Design review of the part built by this model. Coordinates are the model's own, in mm. Face numbers are marked on the shaded views. Give positions to 0.01 mm unless a question says otherwise; leave off trailing zeros. Loops run counter-clockwise (first coordinate to the right, second up) from the corner with the lowest first, then second, coordinate; pieces in that order, holes last. Notation, with made-up numbers: (2.5, 83.5) -> (46.5, 83.5) arc R17 ccw to (46.5, 96.5) -> close; hole circle Ø8 at (18.5, 63.25). An arc over 180 degrees is marked (long way). Use a Markdown table: item, result. Add a question column.
1. Add section B-B (z = 4). State the section outline as (x, y) points (3 decimals).
2. To check wall thickness, follow line 1 (X direction, y = -40.5, z = 4.25); line 2 (Y direction, x = -30.5, z = 2.75); line 3 (X direction, y = 5.5, z = 2.75). State the ranges of each line that lie inside material, in increasing order.
3. Add section C-C (y = 38.5). State the section outline as (x, z) points, and give its area (3 significant figures).
4. Add section A-A (x = 36.5). State the section outline as (y, z) points, and give its area (3 significant figures).
5. Draft analysis for pull direction Y (two halves, no side actions). For the marked faces 1 and 2, state which applies: pulls with the +Y half, pulls with the -Y half, needs draft (parallel to the pull), parting line crosses it, or undercut.
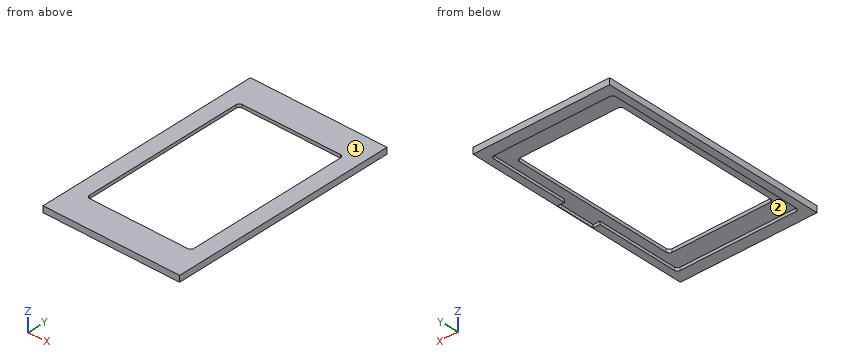
```python
from build123d import *

# Parameters (mm, degrees)
SKETCH1_W           = 140
SKETCH1_H           = 234
BOSS_EXTRUDE1_DEPTH = 6.35
SKETCH2_W           = 107
SKETCH2_H           = 172
CUT_EXTRUDE1_DEPTH  = 137.489276136
FILLET1_R           = 3.175
SKETCH3_W           = 125
SKETCH3_H           = 210
CUT_EXTRUDE2_DEPTH  = 3
FILLET2_R           = 3.175
SKETCH5_W           = 6
SKETCH5_H           = 40
CUT_EXTRUDE4_DEPTH  = 20
SKETCH6_W           = 0.5
SKETCH6_H           = 40
BOSS_EXTRUDE2_DEPTH = 3


with BuildPart() as part:
    # Sketch1 → Boss-Extrude1 (new body)
    with BuildSketch(Plane.XY):
        Rectangle(SKETCH1_W, SKETCH1_H)
    extrude(amount=BOSS_EXTRUDE1_DEPTH)

    # Sketch2 → Cut-Extrude1 (cut, through all)
    with BuildSketch(Plane.XY.offset(6.35)):
        Rectangle(SKETCH2_W, SKETCH2_H)
    extrude(amount=-CUT_EXTRUDE1_DEPTH, mode=Mode.SUBTRACT)

    # Fillet1
    fillet1_edges = [part.edges().sort_by_distance(p)[0] for p in [
        (53.5, 86, 3.175),
        (53.5, -86, 3.175),
        (-53.5, -86, 3.175),
        (-53.5, 86, 3.175),
    ]]
    fillet(fillet1_edges, radius=FILLET1_R)

    # Sketch3 → Cut-Extrude2 (cut)
    with BuildSketch(Plane(origin=(0, 0, 0), x_dir=(-1, 0, 0), z_dir=(0, 0, -1))):
        Rectangle(SKETCH3_W, SKETCH3_H)
    extrude(amount=-CUT_EXTRUDE2_DEPTH, mode=Mode.SUBTRACT)

    # Fillet2
    fillet2_edges = [part.edges().sort_by_distance(p)[0] for p in [
        (-62.5, 105, 1.5),
        (-62.5, -105, 1.5),
        (62.5, -105, 1.5),
        (62.5, 105, 1.5),
    ]]
    fillet(fillet2_edges, radius=FILLET2_R)

    # Sketch5 → Cut-Extrude4 (cut)
    with BuildSketch(Plane(origin=(70, 0, 0), x_dir=(0, 0, -1), z_dir=(1, 0, 0))):
        with Locations((0, 2)):
            Rectangle(SKETCH5_W, SKETCH5_H)
    extrude(amount=-CUT_EXTRUDE4_DEPTH, mode=Mode.SUBTRACT)

    # Sketch6 → Boss-Extrude2 (add)
    with BuildSketch(Plane(origin=(0, 0, 3), x_dir=(-1, 0, 0), z_dir=(0, 0, -1))):
        with Locations((-69.75, 2)):
            Rectangle(SKETCH6_W, SKETCH6_H)
    extrude(amount=BOSS_EXTRUDE2_DEPTH)


solid = part.part
```
Taken from the geometry:
| question | item | result |
|---|---|---|
| 1 | outline | (-70, -117) -> (70, -117) -> (70, 117) -> (-70, 117) -> close; hole (-53.5, -82.825) arc R3.175 ccw to (-50.325, -86) -> (50.325, -86) arc R3.175 ccw to (53.5, -82.825) -> (53.5, 82.825) arc R3.175 ccw to (50.325, 86) -> (-50.325, 86) arc R3.175 ccw to (-53.5, 82.825) -> close |
| 2 | line 1 | x = -70 to -53.5, 53.5 to 70 |
| 2 | line 2 | y = -117 to -105, 105 to 117 |
| 2 | line 3 | x = -70 to -62.5, 69.5 to 70 |
| 3 | outline | (-70, 0) -> (-62.5, 0) -> (-62.5, 3) -> (-53.5, 3) -> (-53.5, 6.35) -> (-70, 6.35) -> close; (53.5, 3) -> (62.5, 3) -> (62.5, 0) -> (70, 0) -> (70, 6.35) -> (53.5, 6.35) -> close |
| 3 | area | 156 mm^2 |
| 4 | outline | (-117, 0) -> (-105, 0) -> (-105, 3) -> (-86, 3) -> (-86, 6.35) -> (-117, 6.35) -> close; (86, 3) -> (105, 3) -> (105, 0) -> (117, 0) -> (117, 6.35) -> (86, 6.35) -> close |
| 4 | area | 280 mm^2 |
| 5 | face 1 | needs draft |
| 5 | face 2 | undercut |
